The listing builds one solid part. Answer for the finished solid, in the listing's coordinates (mm). Face numbers are marked on the shaded views. Give positions to 0.01 mm unless a question says otherwise; leave off trailing zeros. Order: outer loops, then holes, each group sorted by start corner. A loop starts at its lowest first (then second) coordinate and runs counter-clockwise, first axis right, second up. Notation, with made-up numbers: (12.5, -14) -> (50.5, -14) arc R32 ccw to (50.5, 19) -> close; hole circle Ø10 at (25.5, 71.5). An arc over 180 degrees is marked (long way). One line per question, with ' | ' between items. Start each with the question number.
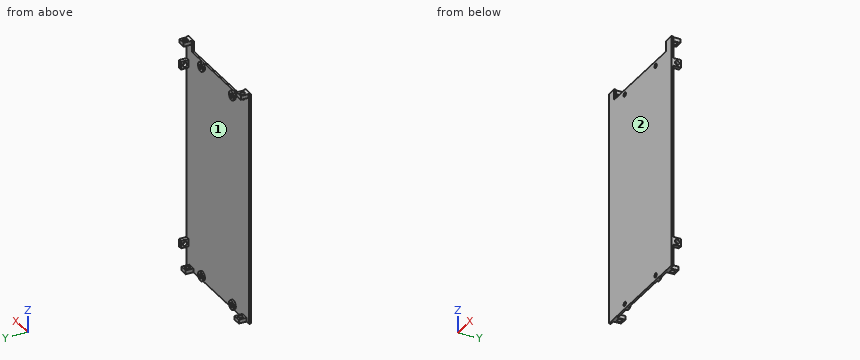
```python
from build123d import *

# Parameters (mm, degrees)
BOSS_EXTRUDE1_DEPTH = 2
SKETCH2_W           = 8
SKETCH2_H           = 4
SKETCH2_W_2         = 4
SKETCH2_H_2         = 8
BOSS_EXTRUDE2_DEPTH = 8
CUT_EXTRUDE1_REACH  = 243.2
SKETCH3_R           = 2.25
CUT_EXTRUDE3_REACH  = 243.2
SKETCH5_R           = 2.25
CUT_EXTRUDE4_REACH  = 123.2
SKETCH6_R           = 2.25
SKETCH7_R           = 4.75
SKETCH7_R_2         = 2.25
BOSS_EXTRUDE3_DEPTH = 4
CUT_EXTRUDE5_REACH  = 6
SKETCH8_R           = 2.25


with BuildPart() as part:
    # Sketch1 → Boss-Extrude1 (new body)
    with BuildSketch(Plane(origin=(0, 0, 0), x_dir=(1, 0, 0), z_dir=(0, 1, 0))):
        Polygon((0.4, 241.6), (121.6, 241.6), (121.6, 0.4), (111.4, 0.4), (111.4, 11.4), (10.6, 11.4), (10.6, 0.4), (0.4, 0.4), align=None)
    extrude(amount=BOSS_EXTRUDE1_DEPTH)

    # Sketch2 → Boss-Extrude2 (add)
    with BuildSketch(Plane(origin=(0, 2, 0), x_dir=(1, 0, 0), z_dir=(0, 1, 0))):
        with Locations((9.5, 239.6)):
            Rectangle(SKETCH2_W, SKETCH2_H)
        with Locations((112.5, 239.6)):
            Rectangle(SKETCH2_W, SKETCH2_H)
        with Locations((5.5, 2.4)):
            Rectangle(SKETCH2_W, SKETCH2_H)
        with Locations((116.5, 2.4)):
            Rectangle(SKETCH2_W, SKETCH2_H)
        with Locations((119.6, 27)):
            Rectangle(SKETCH2_W_2, SKETCH2_H_2)
        with Locations((119.6, 215)):
            Rectangle(SKETCH2_W_2, SKETCH2_H_2)
    extrude(amount=BOSS_EXTRUDE2_DEPTH)

    # Sketch3 → Cut-Extrude1 (cut, up to next)
    with BuildSketch(Plane.XY.offset(-0.4), mode=Mode.PRIVATE) as cut_extrude1_sk1:
        with Locations((5.5, 6)):
            Circle(SKETCH3_R)
    cut_extrude1_tool1 = extrude(cut_extrude1_sk1.sketch, amount=-CUT_EXTRUDE1_REACH, mode=Mode.PRIVATE) & part.part
    add(cut_extrude1_tool1.solids().sort_by_distance((5.5, 6, -0.4))[0], mode=Mode.SUBTRACT)
    # Sketch3 → Cut-Extrude1 (cut, up to next)
    with BuildSketch(Plane.XY.offset(-0.4), mode=Mode.PRIVATE) as cut_extrude1_sk2:
        with Locations((116.5, 6)):
            Circle(SKETCH3_R)
    cut_extrude1_tool2 = extrude(cut_extrude1_sk2.sketch, amount=-CUT_EXTRUDE1_REACH, mode=Mode.PRIVATE) & part.part
    add(cut_extrude1_tool2.solids().sort_by_distance((116.5, 6, -0.4))[0], mode=Mode.SUBTRACT)

    # Sketch5 → Cut-Extrude3 (cut, up to next)
    with BuildSketch(Plane(origin=(0, 0, -241.6), x_dir=(-1, 0, 0), z_dir=(0, 0, -1)), mode=Mode.PRIVATE) as cut_extrude3_sk1:
        with Locations((-112.5, 6)):
            Circle(SKETCH5_R)
    cut_extrude3_tool1 = extrude(cut_extrude3_sk1.sketch, amount=-CUT_EXTRUDE3_REACH, mode=Mode.PRIVATE) & part.part
    add(cut_extrude3_tool1.solids().sort_by_distance((112.5, 6, -241.6))[0], mode=Mode.SUBTRACT)
    # Sketch5 → Cut-Extrude3 (cut, up to next)
    with BuildSketch(Plane(origin=(0, 0, -241.6), x_dir=(-1, 0, 0), z_dir=(0, 0, -1)), mode=Mode.PRIVATE) as cut_extrude3_sk2:
        with Locations((-9.5, 6)):
            Circle(SKETCH5_R)
    cut_extrude3_tool2 = extrude(cut_extrude3_sk2.sketch, amount=-CUT_EXTRUDE3_REACH, mode=Mode.PRIVATE) & part.part
    add(cut_extrude3_tool2.solids().sort_by_distance((9.5, 6, -241.6))[0], mode=Mode.SUBTRACT)

    # Sketch6 → Cut-Extrude4 (cut, up to next)
    with BuildSketch(Plane(origin=(121.6, 0, 0), x_dir=(0, 0, -1), z_dir=(1, 0, 0)), mode=Mode.PRIVATE) as cut_extrude4_sk1:
        with Locations((27, 6)):
            Circle(SKETCH6_R)
    cut_extrude4_tool1 = extrude(cut_extrude4_sk1.sketch, amount=-CUT_EXTRUDE4_REACH, mode=Mode.PRIVATE) & part.part
    add(cut_extrude4_tool1.solids().sort_by_distance((121.6, 6, -27))[0], mode=Mode.SUBTRACT)
    # Sketch6 → Cut-Extrude4 (cut, up to next)
    with BuildSketch(Plane(origin=(121.6, 0, 0), x_dir=(0, 0, -1), z_dir=(1, 0, 0)), mode=Mode.PRIVATE) as cut_extrude4_sk2:
        with Locations((215, 6)):
            Circle(SKETCH6_R)
    cut_extrude4_tool2 = extrude(cut_extrude4_sk2.sketch, amount=-CUT_EXTRUDE4_REACH, mode=Mode.PRIVATE) & part.part
    add(cut_extrude4_tool2.solids().sort_by_distance((121.6, 6, -215))[0], mode=Mode.SUBTRACT)

    # Sketch7 → Boss-Extrude3 (add)
    with BuildSketch(Plane.XZ):
        with Locations((31, -236.6)):
            Circle(SKETCH7_R)
        with Locations((31, -236.6)):
            Circle(SKETCH7_R_2, mode=Mode.SUBTRACT)
        with Locations((31, -16.4)):
            Circle(SKETCH7_R)
        with Locations((31, -16.4)):
            Circle(SKETCH7_R_2, mode=Mode.SUBTRACT)
        with Locations((91, -236.6)):
            Circle(SKETCH7_R)
        with Locations((91, -236.6)):
            Circle(SKETCH7_R_2, mode=Mode.SUBTRACT)
        with Locations((91, -16.4)):
            Circle(SKETCH7_R)
        with Locations((91, -16.4)):
            Circle(SKETCH7_R_2, mode=Mode.SUBTRACT)
    extrude(amount=-BOSS_EXTRUDE3_DEPTH)

    # Sketch8 → Cut-Extrude5 (cut, up to next)
    with BuildSketch(Plane(origin=(0, 4, 0), x_dir=(1, 0, 0), z_dir=(0, 1, 0)), mode=Mode.PRIVATE) as cut_extrude5_sk1:
        with Locations((31, 16.4)):
            Circle(SKETCH8_R)
    cut_extrude5_tool1 = extrude(cut_extrude5_sk1.sketch, amount=-CUT_EXTRUDE5_REACH, mode=Mode.PRIVATE) & part.part
    add(cut_extrude5_tool1.solids().sort_by_distance((31, 4, -16.4))[0], mode=Mode.SUBTRACT)
    # Sketch8 → Cut-Extrude5 (cut, up to next)
    with BuildSketch(Plane(origin=(0, 4, 0), x_dir=(1, 0, 0), z_dir=(0, 1, 0)), mode=Mode.PRIVATE) as cut_extrude5_sk2:
        with Locations((91, 16.4)):
            Circle(SKETCH8_R)
    cut_extrude5_tool2 = extrude(cut_extrude5_sk2.sketch, amount=-CUT_EXTRUDE5_REACH, mode=Mode.PRIVATE) & part.part
    add(cut_extrude5_tool2.solids().sort_by_distance((91, 4, -16.4))[0], mode=Mode.SUBTRACT)
    # Sketch8 → Cut-Extrude5 (cut, up to next)
    with BuildSketch(Plane(origin=(0, 4, 0), x_dir=(1, 0, 0), z_dir=(0, 1, 0)), mode=Mode.PRIVATE) as cut_extrude5_sk3:
        with Locations((31, 236.6)):
            Circle(SKETCH8_R)
    cut_extrude5_tool3 = extrude(cut_extrude5_sk3.sketch, amount=-CUT_EXTRUDE5_REACH, mode=Mode.PRIVATE) & part.part
    add(cut_extrude5_tool3.solids().sort_by_distance((31, 4, -236.6))[0], mode=Mode.SUBTRACT)
    # Sketch8 → Cut-Extrude5 (cut, up to next)
    with BuildSketch(Plane(origin=(0, 4, 0), x_dir=(1, 0, 0), z_dir=(0, 1, 0)), mode=Mode.PRIVATE) as cut_extrude5_sk4:
        with Locations((91, 236.6)):
            Circle(SKETCH8_R)
    cut_extrude5_tool4 = extrude(cut_extrude5_sk4.sketch, amount=-CUT_EXTRUDE5_REACH, mode=Mode.PRIVATE) & part.part
    add(cut_extrude5_tool4.solids().sort_by_distance((91, 4, -236.6))[0], mode=Mode.SUBTRACT)


solid = part.part
```
(1) The part is cut by section C-C on z = -215. Determine the outline of the cut face in (x, y).
(2) The part is cut by section B-B on x = 91. Determine the outline of the cut face in (y, z).
(3) Determine the mould class of the marked faces 1 and 2 for opening direction Z: pulls with the +Z half, pulls with the -Z half, needs draft (parallel to the pull), parting line crosses it, or undercut.
(4) The part is cut by section D-D on y = 6. State how many separate pieces and enclosed holes the cut face has, plus the area to 3 significant figures.
(5) Given P1, Ø7, axis at x = 31, z = -16.4, coming from the +Y side; P2, Ø2.5, axis at y = 6, z = -27, coming from the -X side; P3, Ø5, axis at x = 36.5, z = -105, coming from the +Y side; P4, Ø4.5, axis at y = 5, z = -240, coming from the -X side, each flat-ended and moving along its own axis, determine where each tip first touches the part or whether it passes through.
(6) Consider line 1 (Z direction, x = 90, y = 1.5); line 2 (Y direction, x = 80, z = -174.5); line 3 (Z direction, x = 8.5, y = 9.75). Determine where each line is inside the solid, lowest interval first.
(7) The part is cut by section A-A on z = -16.4. Determine the outline of the cut face in (x, y), plus the area to 3 significant figures.
Result sheet:
1) outline: (0.4, 0) -> (121.6, 0) -> (121.6, 3.75) -> (117.6, 3.75) -> (117.6, 2) -> (0.4, 2) -> close; (117.6, 8.25) -> (121.6, 8.25) -> (121.6, 10) -> (117.6, 10) -> close
2) outline: (0, -241.6) -> (2, -241.6) -> (2, -241.35) -> (4, -241.35) -> (4, -238.85) -> (0, -238.85) -> close; (0, -234.35) -> (4, -234.35) -> (4, -231.85) -> (2, -231.85) -> (2, -21.15) -> (4, -21.15) -> (4, -18.65) -> (0, -18.65) -> close; (0, -14.15) -> (4, -14.15) -> (4, -11.65) -> (2, -11.65) -> (2, -11.4) -> (0, -11.4) -> close
3) face 1: undercut | face 2: needs draft
4) separate pieces: 12 | enclosed holes: 0 | area: 84.0 mm^2
5) P1: stops at y = 4 | P2: passes through | P3: stops at y = 2 | P4: stops at x = 5.5
6) line 1: z = -241.6 to -238.62, -234.58 to -18.42, -14.38 to -11.4 | line 2: y = 0 to 2 | line 3: z = -241.6 to -237.6, -4.4 to -0.4
7) outline: (0.4, 0) -> (28.75, 0) -> (28.75, 4) -> (26.25, 4) -> (26.25, 2) -> (0.4, 2) -> close; (33.25, 0) -> (88.75, 0) -> (88.75, 4) -> (86.25, 4) -> (86.25, 2) -> (35.75, 2) -> (35.75, 4) -> (33.25, 4) -> close; (93.25, 0) -> (121.6, 0) -> (121.6, 2) -> (95.75, 2) -> (95.75, 4) -> (93.25, 4) -> close | area: 244 mm^2
